Solid Edge part; units mm, degrees
sketch "Sketch1" plane through (0, 0, 0) normal (0, -1, 0) x (1, 0, 0)
  line L0 (30, 150) -> (30, 80)
  line L1 (30, 80) -> (30, 60)
  line L2 (40, 50) -> (90, 50)
  line L3 (90, 0) -> (0, 0)
  line L4 (0, 0) -> (-90, 0)
  line L5 (-90, 50) -> (-40, 50)
  line L6 (-30, 60) -> (-30, 80)
  line L7 (-30, 80) -> (-30, 150)
  arc A0 (40, 50) -> (30, 60) centre (40, 60) cw
  arc A1 (90, 50) -> (90, 0) centre (90, 25) cw
  arc A2 (-90, 0) -> (-90, 50) centre (-90, 25) cw
  arc A3 (-40, 50) -> (-30, 60) centre (-40, 60) ccw
  arc A4 (-30, 150) -> (30, 150) centre (0, 150) cw
extrude "Protrusion1" add sketch "Sketch1" against normal blind 30
sketch "Sketch2" plane through (0, 0, 0) normal (0, -1, 0) x (1, 0, 0)
  circle A0 centre (0, 150) radius 30
extrude "ExtrudedProtrusion_2" add sketch "Sketch2" along normal blind 10
sketch "Sketch3" plane through (0, 0, 0) normal (0, -1, 0) x (1, 0, 0)
  circle A0 centre (0, 150) radius 15
extrude "Cutout1" cut sketch "Sketch3" along normal mid plane 60
sketch "Sketch4" plane through (0, 0, 0) normal (0, -1, 0) x (1, 0, 0)
  circle A0 centre (90, 25) radius 10
extrude "Cutout2" cut sketch "Sketch4" along normal mid plane 60
sketch "Sketch5" plane through (0, 0, 0) normal (0, -1, 0) x (1, 0, 0)
  circle A0 centre (-90, 25) radius 10
extrude "ExtrudedCutout_3" cut sketch "Sketch5" along normal mid plane 60
sketch "Sketch6" plane through (0, 0, 0) normal (1, 0, 0) x (0, 1, 0)
  line L0 (0, 80) -> (-75, 50)
  line L1 (-75, 0) -> (0, 0)
  line L2 (0, 0) -> (0, 25)
  line L3 (0, 25) -> (0, 80)
  arc A0 (-75, 0) -> (-75, 50) centre (-75, 25) cw
extrude "ExtrudedProtrusion_4" add sketch "Sketch6" along normal mid plane 60
sketch "Sketch7" plane through (0, 0, 0) normal (1, 0, 0) x (0, 1, 0)
  circle A0 centre (-75, 25) radius 12.5
extrude "ExtrudedCutout_4" cut sketch "Sketch7" along normal mid plane 60
sketch "Sketch8" plane through (0, 0, 0) normal (1, 0, 0) x (0, 1, 0)
  line L0 (0, 80) -> (-75, 50)
  line L1 (0, 25) -> (0, 80)
  line L2 (0, 0) -> (0, 25)
  line L3 (-75, 0) -> (0, 0)
  arc A0 (-75, 0) -> (-75, 50) centre (-75, 25) cw
extrude "ExtrudedCutout_5" cut sketch "Sketch8" along normal mid plane 30
Read the model definition and answer for the solid it produces. Units are mm, in the model's axes. A direction names the side the tool comes from. Give positions to 0.01 mm unless a question says otherwise; leave off trailing zeros. Write each loop counter-clockwise with the first axis right and the second up, starting at its lowest first coordinate (ties: lowest second). Pieces come first, ordered by that corner, then holes. Notation, with made-up numbers: (82.25, 32) - (92.25, 32) arc R10 ccw to (92.25, 40) - close; hole circle Ø8 at (62.25, 19). An arc over 180 degrees is marked (long way). Answer in a Markdown table with one row per item. Add a question column.
Item 1: Determine the mould class of faces 1 (the face through (80, 15, 25)), 2 (the face through (-72, 0, 23)), 3 (the face through (22.395, -77.71, 37.203)) for opening direction Y: pulls with the +Y half, pulls with the -Y half, needs draft (parallel to the pull), parting line crosses it, or undercut.
Item 2: Flat-ended cylindrical pins translate along their axes: P1, Ø1, axis at x = -27.5, y = -58.5, coming from the +Z side; P2, Ø16, axis at x = -90, z = 25, coming from the -Y side; P3, Ø18, axis at x = 7, z = 164, coming from the -Y side; P4, Ø15, axis at x = 75.5, y = 19.5, coming from the +Z side. Find the tip coordinate at first contact, or state that the pin passes through.
Item 3: Section B-B, the plane y = -19.5 is taken. Write down the section's boundary in (x, z).
Item 4: Section A-A, the plane x = 0 is taken. Write down the section's boundary in (y, z).
Item 5: Find the intervals of material crossed by L1, parallel to Z at x = 0, y = 8; L2, parallel to X at y = 7.5, z = 150; L3, parallel to Y at x = -19, z = 25, in increasing order.
Item 6: Section C-C, the plane z = 142 is taken. Write down the section's boundary in (x, y).
Item 7: Section D-D, the plane x = -24.5 is taken. Write down the section's boundary in (y, z), and give its area (3 significant figures).
Item 8: A tool of negligible diameter and unlimited length cuts with its end or side. For faces 4 (the face through (14, -10, 144)), 5 (the face through (-30, -21, 57)), 6 (the face through (-65, 15, 50)), 7 (the face through (15, -40, 31)), from which of +Z, -Z, +X, -X, +Y, -Y can it reach the whole face along a straight path? Write none if from no direction.
Recorded:
| question | item | result |
|---|---|---|
| 1 | face 1 | needs draft |
| 1 | face 2 | pulls with the -Y half |
| 1 | face 3 | undercut |
| 2 | P1 | stops at z = 56.8 |
| 2 | P2 | passes through |
| 2 | P3 | stops at y = -10 |
| 2 | P4 | stops at z = 50 |
| 3 | outline | (-30, 0) - (-15, 0) - (-15, 72.2) - (-30, 72.2) - close; (15, 0) - (30, 0) - (30, 72.2) - (15, 72.2) - close |
| 4 | outline | (-10, 120) - (0, 120) - (0, 0) - (30, 0) - (30, 135) - (-10, 135) - close; (-10, 165) - (30, 165) - (30, 180) - (-10, 180) - close |
| 5 | L1 | z = 0 to 135, 165 to 180 |
| 5 | L2 | x = -30 to -15, 15 to 30 |
| 5 | L3 | y = -100 to -87.5, -62.5 to 30 |
| 6 | outline | (-30, 0) - (-28.91, 0) - (-28.91, -10) - (-12.69, -10) - (-12.69, 30) - (-30, 30) - close; (12.69, -10) - (28.91, -10) - (28.91, 0) - (30, 0) - (30, 30) - (12.69, 30) - close |
| 7 | outline | (-75, 0) - (30, 0) - (30, 167.31) - (-10, 167.31) - (-10, 132.69) - (0, 132.69) - (0, 80) - (-75, 50) arc R25 ccw to start; hole circle Ø25 at (-75, 25) |
| 7 | area | 10,700 mm2 |
| 8 | face 4 | +Z, +X, -X, -Y |
| 8 | face 5 | +Z, -X, -Y |
| 8 | face 6 | +Z, -X, +Y, -Y |
| 8 | face 7 | -Z, -Y |
